Here's how the part is built. I have some questions about the finished solid (model axes, mm). Face numbers are marked on the shaded views. Give positions to 0.01 mm unless a question says otherwise; leave off trailing zeros. Write each loop counter-clockwise with the first axis right and the second up, starting at its lowest first coordinate (ties: lowest second). Pieces come first, ordered by that corner, then holes. Notation, with made-up numbers: (-33.75, -8.5) -> (-20.75, -8.5) arc R18 cw to (-20.75, 10.5) -> close; hole circle Ø5 at (23.25, 52.25). An arc over 180 degrees is marked (long way). Return JSON: item names as keys, results as strings.
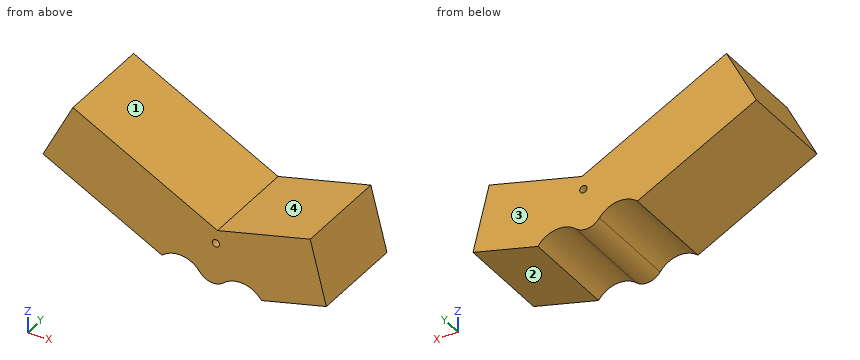
from build123d import *

# Parameters (mm, degrees)
F1_DEPTH = 3.81
F2_R     = 0.1456869123
F3_DEPTH = 3.81
F5_DEPTH = 25.4


with BuildPart() as f1:
    # F0 (on Front) → F1 (new body)
    with BuildSketch(Plane.XZ):
        with BuildLine():
            Line((4.8432132158, 18.5995820194), (-0.7969688229, 21.5169175451))
            Line((-0.7969688229, 21.5169175451), (-1.9639030332, 19.2608447295))
            Line((-1.9639030332, 19.2608447295), (2.6801745949, 16.8587356211))
            ThreePointArc((2.6801745949, 16.8587356211), (3.4526909685, 17.1123534538), (4.1582529007, 16.708266938))
            ThreePointArc((4.1582529007, 16.708266938), (4.5987642694, 16.4524828685), (5.0854991089, 16.6026992195))
            ThreePointArc((5.0854991089, 16.6026992195), (5.8638378577, 16.8378424622), (6.5595735586, 16.4170629629))
            Line((6.5595735586, 16.4170629629), (11.6247636885, 17.7137642129))
            Line((11.6247636885, 17.7137642129), (10.9948318325, 20.1744116595))
            Line((10.9948318325, 20.1744116595), (4.8432132158, 18.5995820194))
        make_face()
    extrude(amount=F1_DEPTH)

    # F2 (on face) → F3 (cut, through all)
    with BuildSketch(Plane.XZ.offset(3.81)):
        with Locations((4.7830365223, 18.0710245049)):
            Circle(F2_R)
    extrude(amount=-F3_DEPTH, mode=Mode.SUBTRACT)

    # F4 (on face) → F5 (cut)
    with BuildSketch(Plane.XZ.offset(3.81)):
        Polygon((11.6247636885, 17.7137642129), (10.9948318325, 20.1744116595), (8.4622367675, 19.5260610345), (9.0921686236, 17.0654135879), align=None)
    extrude(amount=-F5_DEPTH, mode=Mode.SUBTRACT)


solid = f1.part
1. Suppose I cut it at B-B, the plane y = -0.45. List the corners of the cut face in (x, z) for me (1 decimal), and give its area (3 significant figures).
Taken from the geometry:
{"outline": "(-2, 19.3) -> (2.7, 16.9) arc R1 cw to (4.2, 16.7) arc R0.6 ccw to (5.1, 16.6) arc R1 cw to (6.6, 16.4) -> (9.1, 17.1) -> (8.5, 19.5) -> (4.8, 18.6) -> (-0.8, 21.5) -> close; hole circle Ø0.3 at (4.8, 18.1)", "area": "26.0 mm²"}
2. Suppose I cut it at D-D, the plane z = 20.2. List the corners of the cut face in (x, y) for me, and give its area (3 significant figures).
Taken from the geometry:
{"outline": "(-1.48, -3.81) -> (1.75, -3.81) -> (1.75, 0) -> (-1.48, 0) -> close", "area": "12.3 mm²"}
3. If we mould it in two halves opening along X, with no side actions, what happens to the marked faces 1, 2, 3 and 4? For each: released by +X, released by -X, zero draft, split by the parting line, or undercut.
Taken from the geometry:
{"face 1": "undercut", "face 2": "released by +X", "face 3": "zero draft", "face 4": "undercut"}
4. Suppose I cut it at A-A, the plane z = 18.85. List the corners of the cut face in (x, y) for me.
Taken from the geometry:
{"outline": "(-1.17, -3.81) -> (4.36, -3.81) -> (4.36, 0) -> (-1.17, 0) -> close; (5.82, -3.81) -> (8.64, -3.81) -> (8.64, 0) -> (5.82, 0) -> close"}
5. If I drill on line 1 (X direction, y = -2.1, z = 18.1); line 2 (X direction, y = -2.45, z = 18.5); line 3 (X direction, y = -3.45, z = 18.15), over which ranges is the centre line in solid material (lowest first)? Write a range as [from, to].
Taken from the geometry:
{"line 1": "x = [0.28, 4.64], [4.93, 8.83]", "line 2": "x = [-0.49, 8.72]", "line 3": "x = [0.18, 4.66], [4.91, 8.81]"}
6. Suppose I cut it at C-C, the plane x = 7.5. List the corners of the cut face in (y, z) for me, and give its area (3 significant figures).
Taken from the geometry:
{"outline": "(-3.81, 16.66) -> (0, 16.66) -> (0, 19.28) -> (-3.81, 19.28) -> close", "area": "9.99 mm²"}
7. For pin 1 Ø1.5 at (x, y) = (3.5, -2.5) entering from +Z; pin 2 Ø1.5 at (x, y) = (4.5, -3) entering from -Z; pin 3 Ø2 at (x, y) = (7, -3) entering from +Z, each with a flat end and sliding along its axis, tell me the tip position at first contact or that it passes through.
Taken from the geometry:
{"pin 1": "stops at z = 19.68", "pin 2": "stops at z = 16.45", "pin 3": "stops at z = 19.41"}
